from build123d import *

# Parameters (mm, degrees)
SKETCH1_W           = 15
SKETCH1_H           = 50
BOSS_EXTRUDE1_DEPTH = 310
SKETCH2_W           = 60
SKETCH2_H           = 70
BOSS_EXTRUDE2_DEPTH = 2
SKETCH4_R           = 3
CUT_EXTRUDE1_DEPTH  = 2
FILLET1_R           = 6
SKETCH5_R           = 13.5
CUT_EXTRUDE2_DEPTH  = 7
SKETCH6_R           = 11
CUT_EXTRUDE3_DEPTH  = 314.456934841
FILLET2_R           = 6


with BuildPart() as part:
    # Sketch1 → Boss-Extrude1 (new body)
    with BuildSketch(Plane(origin=(0, 0, 0), x_dir=(1, 0, 0), z_dir=(0, 1, 0))):
        Rectangle(SKETCH1_W, SKETCH1_H)
    extrude(amount=BOSS_EXTRUDE1_DEPTH)

    # Sketch2 → Boss-Extrude2 (add)
    with BuildSketch(Plane(origin=(0, 0, 0), x_dir=(-1, 0, 0), z_dir=(0, -1, 0))):
        Rectangle(SKETCH2_W, SKETCH2_H)
    extrude(amount=BOSS_EXTRUDE2_DEPTH)

    # Sketch4 → Cut-Extrude1 (cut)
    with BuildSketch(Plane(origin=(0, 0, 0), x_dir=(1, 0, 0), z_dir=(0, 1, 0))):
        with Locations(Location((20, -25, 0), (0, 0, 270))):
            Circle(SKETCH4_R)
        with Locations(Location((-20, -25, 0), (0, 0, 90))):
            Circle(SKETCH4_R)
        with Locations(Location((-20, 25, 0), (0, 0, 270))):
            Circle(SKETCH4_R)
        with Locations(Location((20, 25, 0), (0, 0, 90))):
            Circle(SKETCH4_R)
    extrude(amount=-CUT_EXTRUDE1_DEPTH, mode=Mode.SUBTRACT)

    # Fillet1
    fillet1_edges = [part.edges().sort_by_distance(p)[0] for p in [
        (-30, -1, 35),
        (-30, -1, -35),
        (30, -1, -35),
        (30, -1, 35),
    ]]
    fillet(fillet1_edges, radius=FILLET1_R)

    # Sketch5 → Cut-Extrude2 (cut)
    with BuildSketch(Plane.ZY.offset(7.5)):
        with Locations((0, 280)):
            Circle(SKETCH5_R)
    extrude(amount=-CUT_EXTRUDE2_DEPTH, mode=Mode.SUBTRACT)

    # Sketch6 → Cut-Extrude3 (cut, through all)
    with BuildSketch(Plane.ZY.offset(0.5)):
        with Locations((0, 280)):
            Circle(SKETCH6_R)
    extrude(amount=-CUT_EXTRUDE3_DEPTH, mode=Mode.SUBTRACT)

    # Fillet2
    fillet2_edges = [part.edges().sort_by_distance(p)[0] for p in [
        (0, 310, 25),
        (0, 310, -25),
    ]]
    fillet(fillet2_edges, radius=FILLET2_R)


solid = part.part
Geometry: final body of the model. Coordinates: model frame, mm. A direction names the side the tool comes from. Give positions to 0.01 mm unless a question says otherwise; leave off trailing zeros. Order: outer loops, then holes, each group sorted by start corner. A loop starts at its lowest first (then second) coordinate and runs counter-clockwise, first axis right, second up. Notation, with made-up numbers: (-16, -6) -> (25, -6) arc R24 ccw to (25, 22) -> close; hole circle Ø5 at (84.25, -36.5). An arc over 180 degrees is marked (long way). Write each question's results on one line, items separated by ' | '.
1) Cut plane A-A (x = 4). Output: boundary loops of the cut face in (y, z).
Geometry says:
outline: (-2, -35) -> (0, -35) -> (0, -25) -> (304, -25) arc R6 ccw to (310, -19) -> (310, 19) arc R6 ccw to (304, 25) -> (0, 25) -> (0, 35) -> (-2, 35) -> close; hole circle Ø22 at (280, 0)
2) Cut plane B-B (z = 0). Output: boundary loops of the cut face in (x, y).
Geometry says:
outline: (-30, -2) -> (30, -2) -> (30, 0) -> (7.5, 0) -> (7.5, 269) -> (-0.5, 269) -> (-0.5, 266.5) -> (-7.5, 266.5) -> (-7.5, 0) -> (-30, 0) -> close; (-7.5, 293.5) -> (-0.5, 293.5) -> (-0.5, 291) -> (7.5, 291) -> (7.5, 310) -> (-7.5, 310) -> close
3) Cut plane D-D (x = 20). Output: boundary loops of the cut face in (y, z).
Geometry says:
outline: (-2, -35) -> (0, -35) -> (0, -28) -> (-2, -28) -> close; (-2, -22) -> (0, -22) -> (0, 22) -> (-2, 22) -> close; (-2, 28) -> (0, 28) -> (0, 35) -> (-2, 35) -> close
4) Set-up query: faces 1 (the face through (-7.5, 153, 0)), 2 (the face through (0, 150, -25)), 3 (the face through (0, 150, 25)), 4 (the face through (7.5, 153, 0)). Return all of +Z, -Z, +X, -X, +Y, -Y with unobstructed straight access to the full face (end or side cutting, diameter ignored); none if empty.
Geometry says:
face 1: +Z, -Z, -X, +Y | face 2: -Z, +X, -X, +Y | face 3: +Z, +X, -X, +Y | face 4: +Z, -Z, +X, +Y
5) Cut plane C-C (y = 280). Output: boundary loops of the cut face in (x, z), and give its area (3 significant figures).
Geometry says:
outline: (-7.5, -25) -> (7.5, -25) -> (7.5, -11) -> (-0.5, -11) -> (-0.5, -13.5) -> (-7.5, -13.5) -> close; (-7.5, 13.5) -> (-0.5, 13.5) -> (-0.5, 11) -> (7.5, 11) -> (7.5, 25) -> (-7.5, 25) -> close | area: 385 mm²
6) First-contact query: pin 1 Ø20 at (y, z) = (280, 0) entering from -X; pin 2 Ø25 at (y, z) = (120, 11.5) entering from +X; pin 3 Ø12 at (y, z) = (236, 11.5) entering from -X; pin 4 Ø4.5 at (x, y) = (-3.5, 148) entering from +Z. Flat tips, straight axial feed; report the tip coordinate or a pass-through.
Geometry says:
pin 1: passes through | pin 2: stops at x = 7.5 | pin 3: stops at x = -7.5 | pin 4: stops at z = 25
7) Line query: line 1 along X through (y, z) = (-1, 25); line 2 along Y through (x, z) = (-4.75, 0); line 3 along Z through (x, y) = (-4, 124). Output: solid intervals per line, ascending.
Geometry says:
line 1: x = -30 to -23, -17 to 17, 23 to 30 | line 2: y = -2 to 266.5, 293.5 to 310 | line 3: z = -25 to 25
8) Draft query along Y for faces 5 (the face through (22.93, -0.99, -24.35)), 6 (the face through (0.105, 308.196, 23.289)), 7 (the face through (-0.5, 270, -5)). Return one class per face: released by +Y, released by -Y, zero draft, split by the parting line, or undercut.
Geometry says:
face 5: zero draft | face 6: released by +Y | face 7: undercut
